Geometry: final body of the model. Coordinates: model frame, mm. Face numbers are marked on the shaded views. A direction names the side the tool comes from. Give positions to 0.01 mm unless a question says otherwise; leave off trailing zeros. Loops run counter-clockwise (first coordinate to the right, second up) from the corner with the lowest first, then second, coordinate; pieces in that order, holes last. Notation, with made-up numbers: (19, 63.5) - (56, 63.5) arc R35 cw to (56, 95.5) - close; hole circle Ø8 at (87.25, -20). An arc over 180 degrees is marked (long way). Use one line per item in the form item = value.
```python
from build123d import *

# Parameters (mm, degrees)
F1_DEPTH = 19.05
F3_DEPTH = 31.17521
F5_DEPTH = 22.95972
F7_DEPTH = 30.07307


with BuildPart() as f1:
    # F0 (on Front) → F1 (new body)
    with BuildSketch(Plane.XZ):
        with BuildLine():
            Line((18.993197, 27.558638), (-31.806803, 27.558638))
            Line((-31.806803, 27.558638), (-31.806803, 21.208638))
            ThreePointArc((-31.806803, 21.208638), (-27.044303, 16.446138), (-22.281803, 21.208638))
            Line((-22.281803, 21.208638), (6.293197, 21.208638))
            Line((6.293197, 21.208638), (6.293197, 8.508638))
            Line((6.293197, 8.508638), (18.993197, 8.508638))
            Line((18.993197, 8.508638), (18.993197, 27.558638))
        make_face()
    extrude(amount=F1_DEPTH)

    # F2 (on face) → F3 (cut)
    with BuildSketch(Plane.XY.offset(27.558638)):
        with BuildLine():
            Line((-19.155291, -7.938241), (-19.058462, -7.938236))
            ThreePointArc((-19.058462, -7.938236), (-19.106877, -7.9375), (-19.155291, -7.938241))
        make_face()
        with BuildLine():
            Line((-3.231877, -7.9375), (-19.058462, -7.938236))
            Line((-19.058462, -7.938236), (-19.155291, -7.938241))
            ThreePointArc((-19.155291, -7.938241), (-20.694118, -9.549247), (-19.106803, -11.1125))
            Line((-19.106803, -11.1125), (-3.231803, -11.1125))
            ThreePointArc((-3.231803, -11.1125), (-1.644303, -9.524963), (-3.231877, -7.9375))
        make_face()
    extrude(amount=-F3_DEPTH, mode=Mode.SUBTRACT)

    # F4 (on face) → F5 (cut)
    with BuildSketch(Plane(origin=(0, 0, 0), x_dir=(-1, 0, 0), z_dir=(0, 1, 0))):
        Polygon((-6.293197, 8.508638), (-6.293197, 11.683638), (-9.526091, 8.508638), align=None)
    extrude(amount=-F5_DEPTH, mode=Mode.SUBTRACT)

    # F6 (on face) → F7 (cut)
    with BuildSketch(Plane.XZ.offset(19.05)):
        Polygon((18.993197, 8.508638), (18.993197, 11.683638), (15.875054, 8.508638), align=None)
    extrude(amount=-F7_DEPTH, mode=Mode.SUBTRACT)


solid = f1.part
```
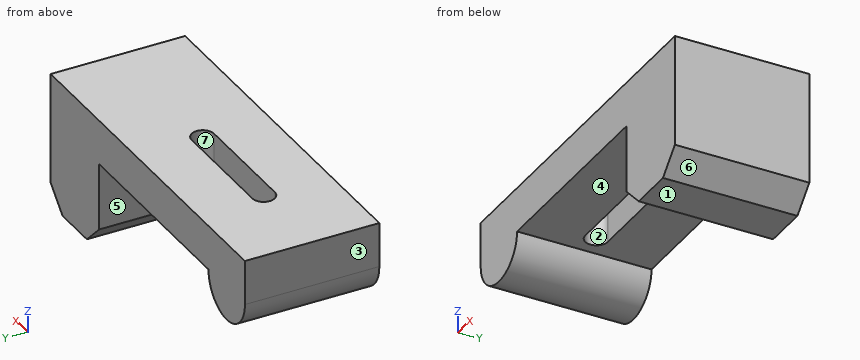
(1) Pull-direction query (X, two-part tool) for the marked faces 1, 2, 3 and 4; classes: released by +X, released by -X, zero draft, split by the parting line, or undercut.
Solution:
face_1 = zero draft
face_2 = undercut
face_3 = released by -X
face_4 = undercut
(2) Material intervals for L1, parallel to Y at x = -8, z = 23; L2, parallel to Z at x = 2, y = -11.5; L3, parallel to X at y = -9.5, z = 21.75, sorted ascending. Write a range as from..to.
Solution:
L1 = -19.05..-11.11, -7.94..0
L2 = 21.21..27.56
L3 = -31.81..-20.69, -1.64..18.99
(3) Cut plane C-C (x = -13). Return the cut outline in (y, z).
Solution:
outline = (-19.05, 21.21) - (-11.11, 21.21) - (-11.11, 27.56) - (-19.05, 27.56) - close; (-7.94, 21.21) - (0, 21.21) - (0, 27.56) - (-7.94, 27.56) - close
(4) Cut plane D-D (z = 17.75). Return the cut outline in (x, y), plus the area to 3 significant figures.
Solution:
outline = (-30.32, -19.05) - (-23.77, -19.05) - (-23.77, 0) - (-30.32, 0) - close; (6.29, -19.05) - (18.99, -19.05) - (18.99, 0) - (6.29, 0) - close
area = 367 mm2
(5) Pin query (flat end, axial travel): P1, Ø1.5, axis at x = -1, y = -13.5, coming from the -Z side; P2, Ø7.5, axis at y = -7.5, z = 15, coming from the -X side. Return the tip coordinate at first contact, or that it passes through.
Solution:
P1 = 21.21
P2 = -31.12
(6) Access query for the marked faces 5, 6 and 7. Directions: +Z, -Z, +X, -X, +Y, -Y. A direction counts if a zero-diameter tool reaches every point of the face in a straight line with its end or side. Return the directions, or none.
Solution:
face_5 = -Z, +Y, -Y
face_6 = -Z, +X, +Y, -Y
face_7 = +Z, -Z
(7) Cut plane B-B (y = -15). Return the cut outline in (x, z) (1 decimal).
Solution:
outline = (-31.8, 21.2) arc R4.8 ccw to (-22.3, 21.2) - (6.3, 21.2) - (6.3, 11.7) - (9.5, 8.5) - (15.9, 8.5) - (19, 11.7) - (19, 27.6) - (-31.8, 27.6) - close
